The model under review builds one solid part; all positions refer to its coordinate system, in mm. A direction names the side the tool comes from. Coordinates: 2 decimals unless noted, no trailing zeros. Write each loop counter-clockwise with the first axis right and the second up, starting at its lowest first coordinate (ties: lowest second). Pieces come first, ordered by that corner, then holes.
```python
from build123d import *

# Parameters (mm, degrees)
SKETCH1_W           = 18.7
SKETCH1_H           = 3.2
BOSS_EXTRUDE1_DEPTH = 6.35
CUT_EXTRUDE1_DEPTH  = 6.35
BOSS_EXTRUDE2_DEPTH = 6.35
SKETCH4_W           = 25
SKETCH4_H           = 25
BOSS_EXTRUDE3_DEPTH = 6.35


with BuildPart() as part:
    # Sketch1 → Boss-Extrude1 (new body)
    with BuildSketch(Plane(origin=(0, 0, 0), x_dir=(1, 0, 0), z_dir=(0, 1, 0))):
        Polygon((40, -69.282032303), (80, 0), (40, 69.282032303), (-40, 69.282032303), (-80, 0), (-40, -69.282032303), align=None)
        Polygon((-68.56846467, 6.6), (-59.21846467, -9.594675051), (-61.989745962, -11.194675051), (-71.339745962, 5), align=None, mode=Mode.SUBTRACT)
        Polygon((-31.339745962, -64.282032303), (-28.56846467, -62.682032303), (-37.91846467, -46.487357252), (-40.689745962, -48.087357252), align=None, mode=Mode.SUBTRACT)
        Polygon((28.56846467, -62.682032303), (37.91846467, -46.487357252), (40.689745962, -48.087357252), (31.339745962, -64.282032303), align=None, mode=Mode.SUBTRACT)
        Polygon((71.339745962, 5), (68.56846467, 6.6), (59.21846467, -9.594675051), (61.989745962, -11.194675051), align=None, mode=Mode.SUBTRACT)
        with Locations((30.65, 57.682032303)):
            Rectangle(SKETCH1_W, SKETCH1_H, mode=Mode.SUBTRACT)
        with Locations((-30.65, 57.682032303)):
            Rectangle(SKETCH1_W, SKETCH1_H, mode=Mode.SUBTRACT)
    extrude(amount=BOSS_EXTRUDE1_DEPTH)

    # Sketch2 → Cut-Extrude1 (cut)
    with BuildSketch(Plane(origin=(0, 6.35, 0), x_dir=(1, 0, 0), z_dir=(0, 1, 0))):
        Polygon((-59.215390309, 0), (-29.607695155, 51.282032303), (29.607695155, 51.282032303), (59.215390309, 0), (29.607695155, -51.282032303), (-29.607695155, -51.282032303), align=None)
    extrude(amount=-CUT_EXTRUDE1_DEPTH, mode=Mode.SUBTRACT)

    # Sketch3 → Boss-Extrude2 (add)
    with BuildSketch(Plane(origin=(0, 6.35, 0), x_dir=(1, 0, 0), z_dir=(0, 1, 0))):
        Polygon((-6, -3.464101615), (-6, -51.282032303), (6, -51.282032303), (6, -3.464101615), (3, -5.196152423), (0, 0), (-3, -5.196152423), align=None)
        Polygon((6, 0), (6, -3.464101615), (47.411542732, 20.444863729), (41.411542732, 30.837168574), (0, 6.92820323), (3, 5.196152423), (0, 0), align=None)
        Polygon((-47.411542732, 20.444863729), (-6, -3.464101615), (-6, 0), (0, 0), (-3, 5.196152423), (0, 6.92820323), (-41.411542732, 30.837168574), align=None)
        Polygon((-3, 5.196152423), (0, 0), (3, 5.196152423), (0, 6.92820323), align=None)
        Polygon((3, -5.196152423), (6, -3.464101615), (6, 0), (0, 0), align=None)
        Polygon((-6, 0), (-6, -3.464101615), (-3, -5.196152423), (0, 0), align=None)
    extrude(amount=-BOSS_EXTRUDE2_DEPTH)

    # Sketch4 → Boss-Extrude3 (add)
    with BuildSketch(Plane(origin=(0, 6.35, 0), x_dir=(1, 0, 0), z_dir=(0, 1, 0))):
        Rectangle(SKETCH4_W, SKETCH4_H)
    extrude(amount=-BOSS_EXTRUDE3_DEPTH)


solid = part.part
```
Item 1: Take a section at C-C, the plane z = -33.5. Write out the cut boundary in (x, y), plus the area to 3 significant figures.
Solved:
outline: (-60.66, 0) - (-39.87, 0) - (-39.87, 6.35) - (-60.66, 6.35) - close; (39.87, 0) - (60.66, 0) - (60.66, 6.35) - (39.87, 6.35) - close
area: 264 mm2
Item 2: To check wall thickness, follow line 1 along X through (y, z) = (0.75, -3); line 2 along Z through (x, y) = (-30, 5.75); line 3 along X through (y, z) = (2.5, 38). State the ranges of each line that lie inside material, in increasing order.
Solved:
line 1: x = -78.27 to -70.19, -66.49 to -57.48, -17.2 to 17.2, 57.48 to 66.49, 70.19 to 78.27
line 2: z = -69.28 to -59.28, -56.08 to -50.6, -24.25 to -10.39, 50.6 to 60.2, 63.51 to 69.28
line 3: x = -58.06 to -37.28, -6 to 6, 37.28 to 58.06
Item 3: For pin 1 (3.5 mm diameter, centred on y = 1.5, z = -57.5, fed in from +X); pin 2 (1.5 mm diameter, centred on y = 2, z = -26.5, fed in from -X); pin 3 (1 mm diameter, centred on y = 4, z = -57, fed in from +X); pin 4 (1 mm diameter, centred on x = 13.5, z = -4.5, fed in from -Y), all flat-tipped, find the tip position at first contact; note any pin that passes through.
Solved:
pin 1: stops at x = 47.81
pin 2: stops at x = -65.13
pin 3: stops at x = 47.38
pin 4: stops at y = 0
Item 4: Take a section at B-B, the plane x = -66. Write out the cut boundary in (y, z).
Solved:
outline: (0, -24.25) - (6.35, -24.25) - (6.35, -2.15) - (0, -2.15) - close; (0, 4.25) - (6.35, 4.25) - (6.35, 24.25) - (0, 24.25) - close
Item 5: Take a section at A-A, the plane z = 43.5. Write out the cut boundary in (x, y).
Solved:
outline: (-54.89, 0) - (-34.1, 0) - (-34.1, 6.35) - (-54.89, 6.35) - close; (-6, 0) - (6, 0) - (6, 6.35) - (-6, 6.35) - close; (34.1, 0) - (54.89, 0) - (54.89, 6.35) - (34.1, 6.35) - close
Item 6: Mouldability with a two-part tool opening along Z and no side actions: class faces 1 (the face through (-1, 0, -1)), 2 (the face through (-31, 3, -59.282)), 3 (the face through (1, 3, -69.282)) as pulls with the +Z half, pulls with the -Z half, needs draft (parallel to the pull), parting line crosses it, or undercut.
Solved:
face 1: needs draft
face 2: undercut
face 3: pulls with the -Z half
Item 7: Take a section at D-D, the plane y = 1.75. Count the separate pieces of the cut face and the enclosed holes in it, plus the area to 3 significant figures.
Solved:
separate pieces: 1
enclosed holes: 9
area: 9,140 mm2
Item 8: Machinability: for faces 4 (the face through (-1, 3, 69.282)), 5 (the face through (36.08, 3.13, 56.07)), which of the approach directions +Z, -Z, +X, -X, +Y, -Y give a long, thin tool a straight path to every point of the face, cutting with its end or side? Answer none if there is none.
Solved:
face 4: +Z, +X, -X, +Y, -Y
face 5: +Y, -Y
